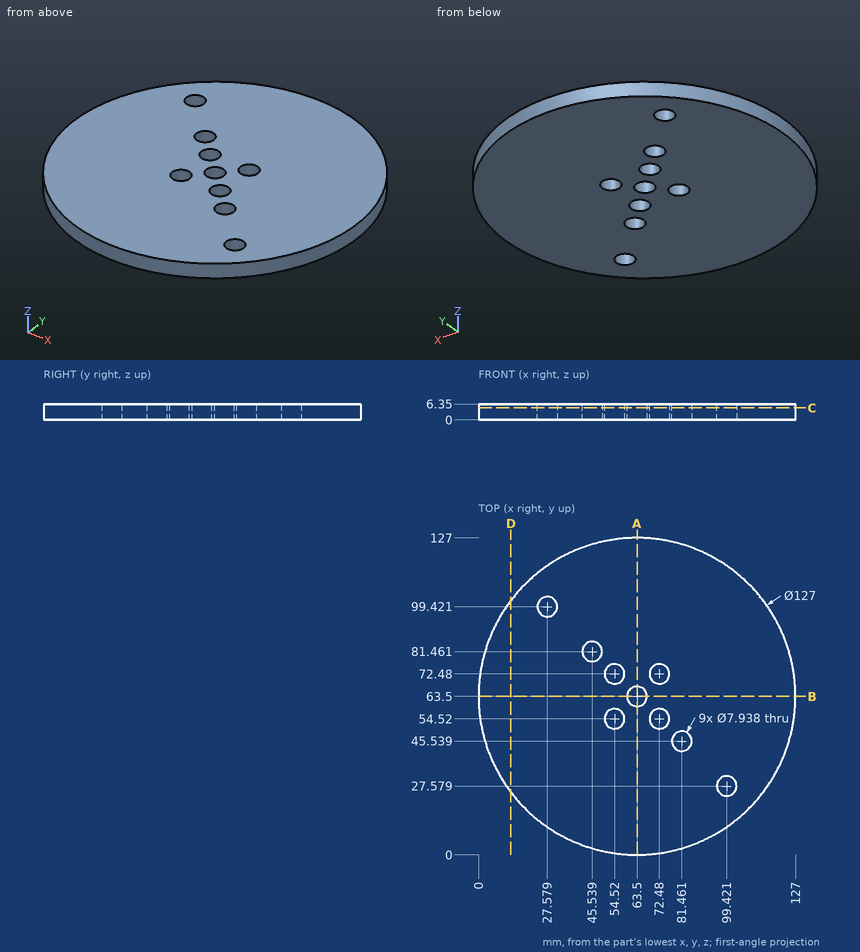
Verification items for this drawing (mm, ordinates from the low corner). Coordinates: 2 decimals unless noted, no trailing zeros. Loops run counter-clockwise (first coordinate to the right, second up) from the corner with the lowest first, then second, coordinate; pieces in that order, holes last. Notation, with made-up numbers: (8, 23) - (52, 23) arc R28 cw to (52, 55) - close; hole circle Ø9 at (27.5, 6.5). An arc over 180 degrees is marked (long way). One line per item, written item: value. Start each with the question number.
(1) Cross-section at D-D on x = 13. Enter the section's corners in (y, z), plus the area to 3 significant figures.
(2) Cross-section at A-A on x = 63.5. Enter the section's corners in (y, z).
(3) Cross-section at C-C on z = 4.75. Count the separate pieces of the cut face and the enclosed holes in it, plus the area to 3 significant figures.
(4) Material ranges on line 1 (X direction, y = 55, z = 0.5); line 2 (X direction, y = 54, z = 0.5) (1 decimal); line 3 (Y direction, x = 25, z = 3) (1 decimal), recorded low to high. Write a range as [from, to].
Results below:
1. outline: (25, 0) - (102, 0) - (102, 6.35) - (25, 6.35) - close
1. area: 489 mm2
2. outline: (0, 0) - (59.53, 0) - (59.53, 6.35) - (0, 6.35) - close; (67.47, 0) - (127, 0) - (127, 6.35) - (67.47, 6.35) - close
3. separate pieces: 1
3. enclosed holes: 9
3. area: 12,200 mm2
4. line 1: x = [0.57, 50.58], [58.46, 68.54], [76.42, 126.43]
4. line 2: x = [0.7, 50.6], [58.5, 68.5], [76.4, 126.3]
4. line 3: y = [13, 96.4], [102.4, 114]
